Can you work these out from the model? Positions are in its coordinate system, mm. A direction names the side the tool comes from. Round coordinates to 2 decimals unless told otherwise and drop trailing zeros. Loops run counter-clockwise (first coordinate to the right, second up) from the corner with the lowest first, then second, coordinate; pieces in that order, holes last. Notation, with made-up numbers: (-17.75, 65) -> (10.25, 65) arc R9 cw to (10.25, 73) -> close; hole circle Ø11 at (41, 88.5). An arc over 180 degrees is marked (long way). Write each question's results on one line, items separated by ' | '.
from build123d import *

# Parameters (mm, degrees)
F0_W         = 111.7644011974
F0_H         = 111.7644011974
F1_DEPTH     = 55.88
F2_R         = 55.8021322807
F3_R         = 55.8038
F5_T1_DEPTH  = 139.6679689167
F5_T3_DEPTH  = 0.1568011974
F5_T5_DEPTH  = 0.1524
F5_T7_DEPTH  = 139.6679689167
F5_T9_DEPTH  = 0.1568011974
F5_S13_W     = 56.919876
F5_S13_H     = 56.919876
F5_T14_DEPTH = 56.919876
F5_S19_W     = 56.919876
F5_S19_H     = 56.919876
F5_T20_DEPTH = 56.919876
F5_S25_W     = 56.919876
F5_S25_H     = 56.919876
F5_T26_DEPTH = 56.919876
F5_S31_W     = 56.919876
F5_S31_H     = 56.919876
F5_T32_DEPTH = 56.919876
F5_T36_ANGLE = 90
F5_T38_ANGLE = 90
F5_T40_ANGLE = 90
F5_T42_ANGLE = 90
F6_R         = 56.7270748454
F7_DEPTH     = 4.826


# Not quite as in the source:
# - a fillet or chamfer that OpenCascade refuses, or shapes differently, is made with other operations: its cross-section is extruded or revolved along the edge and cut away or added
# - a feature of the source that left no trace in its solid (it failed there, or was rolled back) is left out


with BuildPart() as f1:
    # F0 (on Front) → F1 (new body, symmetric)
    with BuildSketch(Plane.XZ):
        with Locations((-0.1386664808, 0)):
            Rectangle(F0_W, F0_H)
    extrude(amount=F1_DEPTH, both=True)

    # F2
    f2_edges = [f1.edges().sort_by_distance(p)[0] for p in [
        (-56.020867, 0, 55.882201),
    ]]
    fillet(f2_edges, radius=F2_R)

    # F3
    f3_edges = [f1.edges().sort_by_distance(p)[0] for p in [
        (55.743534, 0, 55.882201),
    ]]
    fillet(f3_edges, radius=F3_R)

    # F5: fillet of radius 55.8038 on 10 edges, made by hand

    # F5_s2 → F5_t1 (cut)
    with BuildSketch(Plane.YZ.offset(-139.7282347988)):
        with BuildLine():
            ThreePointArc((0.0762, 55.8822005987), (39.535445396, 39.5376459947), (55.88, 0.0784005987))
            Line((55.88, 0.0784005987), (56.996076, 0.0784005987))
            Line((56.996076, 0.0784005987), (56.996076, 56.9982765987))
            Line((56.996076, 56.9982765987), (0.0762, 56.9982765987))
            Line((0.0762, 56.9982765987), (0.0762, 55.8822005987))
        make_face()
        with BuildLine():
            ThreePointArc((-0.0762, 55.8822005987), (-39.535445396, 39.5376459947), (-55.88, 0.0784005987))
            Line((-55.88, 0.0784005987), (-56.996076, 0.0784005987))
            Line((-56.996076, 0.0784005987), (-56.996076, 56.9982765987))
            Line((-56.996076, 56.9982765987), (-0.0762, 56.9982765987))
            Line((-0.0762, 56.9982765987), (-0.0762, 55.8822005987))
        make_face()
    extrude(amount=F5_T1_DEPTH, mode=Mode.SUBTRACT)

    # F5_s4 → F5_t3 (cut)
    with BuildSketch(Plane.YZ.offset(-0.2170670795)):
        with BuildLine():
            ThreePointArc((55.88, -0.0784005987), (39.535445396, -39.5376459947), (0.0762, -55.8822005987))
            Line((0.0762, -55.8822005987), (0.0762, -56.9982765987))
            Line((0.0762, -56.9982765987), (56.996076, -56.9982765987))
            Line((56.996076, -56.9982765987), (56.996076, -0.0784005987))
            Line((56.996076, -0.0784005987), (55.88, -0.0784005987))
        make_face()
        with BuildLine():
            ThreePointArc((-55.88, -0.0784005987), (-39.535445396, -39.5376459947), (-0.0762, -55.8822005987))
            Line((-0.0762, -55.8822005987), (-0.0762, -56.9982765987))
            Line((-0.0762, -56.9982765987), (-56.996076, -56.9982765987))
            Line((-56.996076, -56.9982765987), (-56.996076, -0.0784005987))
            Line((-56.996076, -0.0784005987), (-55.88, -0.0784005987))
        make_face()
    extrude(amount=F5_T3_DEPTH, mode=Mode.SUBTRACT)

    # F5_s6 → F5_t5 (cut)
    with BuildSketch(Plane.XZ.offset(-0.0762)):
        with BuildLine():
            ThreePointArc((55.7435341179, -0.0784005987), (39.3989795139, -39.5376459947), (-0.0602658821, -55.8822005987))
            Line((-0.0602658821, -55.8822005987), (-0.0602658821, -56.9982765987))
            Line((-0.0602658821, -56.9982765987), (56.8596101179, -56.9982765987))
            Line((56.8596101179, -56.9982765987), (56.8596101179, -0.0784005987))
            Line((56.8596101179, -0.0784005987), (55.7435341179, -0.0784005987))
        make_face()
        with BuildLine():
            ThreePointArc((-56.0208670795, -0.0784005987), (-39.6763124755, -39.5376459947), (-0.2170670795, -55.8822005987))
            Line((-0.2170670795, -55.8822005987), (-0.2170670795, -56.9982765987))
            Line((-0.2170670795, -56.9982765987), (-57.1369430795, -56.9982765987))
            Line((-57.1369430795, -56.9982765987), (-57.1369430795, -0.0784005987))
            Line((-57.1369430795, -0.0784005987), (-56.0208670795, -0.0784005987))
        make_face()
    extrude(amount=F5_T5_DEPTH, mode=Mode.SUBTRACT)

    # F5_s8 → F5_t7 (cut)
    with BuildSketch(Plane.XY.offset(-0.0784005987)):
        with BuildLine():
            ThreePointArc((-0.2170670795, -55.88), (-39.6763124755, -39.535445396), (-56.0208670795, -0.0762))
            Line((-56.0208670795, -0.0762), (-57.1369430795, -0.0762))
            Line((-57.1369430795, -0.0762), (-57.1369430795, -56.996076))
            Line((-57.1369430795, -56.996076), (-0.2170670795, -56.996076))
            Line((-0.2170670795, -56.996076), (-0.2170670795, -55.88))
        make_face()
        with BuildLine():
            ThreePointArc((-0.2170670795, 55.88), (-39.6763124755, 39.535445396), (-56.0208670795, 0.0762))
            Line((-56.0208670795, 0.0762), (-57.1369430795, 0.0762))
            Line((-57.1369430795, 0.0762), (-57.1369430795, 56.996076))
            Line((-57.1369430795, 56.996076), (-0.2170670795, 56.996076))
            Line((-0.2170670795, 56.996076), (-0.2170670795, 55.88))
        make_face()
    extrude(amount=F5_T7_DEPTH, mode=Mode.SUBTRACT)

    # F5_s10 → F5_t9 (cut)
    with BuildSketch(Plane.XY.offset(-0.0784005987)):
        with BuildLine():
            ThreePointArc((-0.0602658821, -55.88), (39.3989795139, -39.535445396), (55.7435341179, -0.0762))
            Line((55.7435341179, -0.0762), (56.8596101179, -0.0762))
            Line((56.8596101179, -0.0762), (56.8596101179, -56.996076))
            Line((56.8596101179, -56.996076), (-0.0602658821, -56.996076))
            Line((-0.0602658821, -56.996076), (-0.0602658821, -55.88))
        make_face()
        with BuildLine():
            ThreePointArc((-0.0602658821, 55.88), (39.3989795139, 39.535445396), (55.7435341179, 0.0762))
            Line((55.7435341179, 0.0762), (56.8596101179, 0.0762))
            Line((56.8596101179, 0.0762), (56.8596101179, 56.996076))
            Line((56.8596101179, 56.996076), (-0.0602658821, 56.996076))
            Line((-0.0602658821, 56.996076), (-0.0602658821, 55.88))
        make_face()
    extrude(amount=F5_T9_DEPTH, mode=Mode.SUBTRACT)


with BuildPart() as f5_tool12:
    # F5_s13 → F5_t14 (new body)
    with BuildSketch(Plane.XZ.offset(-0.0762)):
        with Locations((-28.6770050795, -28.5383385987)):
            Rectangle(F5_S13_W, F5_S13_H)
    extrude(amount=-F5_T14_DEPTH)

    # F5_s15 → F5_t16 (revolve, cut)
    with BuildSketch(Plane(origin=(-0.2170670795, 0.0762, -0.0784005987), x_dir=(0.7071067812, 0, 0.7071067812), z_dir=(-0.7071067812, 0, 0.7071067812))):
        with BuildLine():
            ThreePointArc((0, -55.8038), (55.8038, 0), (0, 55.8038))
            Line((0, 55.8038), (0, -55.8038))
        make_face()
    revolve(axis=Axis((-0.2170670795, 0.0762, -0.0784005987), (0, 1, 0)), mode=Mode.SUBTRACT)


with BuildPart() as f1_1:
    add(f1.part)

    # F5_t11: cut F5_tool12
    add(f5_tool12.part, mode=Mode.SUBTRACT)


with BuildPart() as f5_tool18:
    # F5_s19 → F5_t20 (new body)
    with BuildSketch(Plane.XZ.offset(-0.0762)):
        with Locations((28.3996721179, -28.5383385987)):
            Rectangle(F5_S19_W, F5_S19_H)
    extrude(amount=-F5_T20_DEPTH)

    # F5_s21 → F5_t22 (revolve, cut)
    with BuildSketch(Plane(origin=(-0.0602658821, 0.0762, -0.0784005987), x_dir=(-0.7071067812, 0, 0.7071067812), z_dir=(-0.7071067812, 0, -0.7071067812))):
        with BuildLine():
            ThreePointArc((0, -55.8038), (55.8038, 0), (0, 55.8038))
            Line((0, 55.8038), (0, -55.8038))
        make_face()
    revolve(axis=Axis((-0.0602658821, 0.0762, -0.0784005987), (0, 1, 0)), mode=Mode.SUBTRACT)


with BuildPart() as f1_2:
    add(f1_1.part)

    # F5_t17: cut F5_tool18
    add(f5_tool18.part, mode=Mode.SUBTRACT)


with BuildPart() as f5_tool24:
    # F5_s25 → F5_t26 (new body)
    with BuildSketch(Plane.XZ.offset(0.0762)):
        with Locations((-28.6770050795, -28.5383385987)):
            Rectangle(F5_S25_W, F5_S25_H)
    extrude(amount=F5_T26_DEPTH)

    # F5_s27 → F5_t28 (revolve, cut)
    with BuildSketch(Plane(origin=(-0.2170670795, -0.0762, -0.0784005987), x_dir=(0.7071067812, 0, 0.7071067812), z_dir=(0.7071067812, 0, -0.7071067812))):
        with BuildLine():
            ThreePointArc((0, -55.8038), (55.8038, 0), (0, 55.8038))
            Line((0, 55.8038), (0, -55.8038))
        make_face()
    revolve(axis=Axis((-0.2170670795, -0.0762, -0.0784005987), (0, -1, 0)), mode=Mode.SUBTRACT)


with BuildPart() as f1_3:
    add(f1_2.part)

    # F5_t23: cut F5_tool24
    add(f5_tool24.part, mode=Mode.SUBTRACT)


with BuildPart() as f5_tool30:
    # F5_s31 → F5_t32 (new body)
    with BuildSketch(Plane.XZ.offset(0.0762)):
        with Locations((28.3996721179, -28.5383385987)):
            Rectangle(F5_S31_W, F5_S31_H)
    extrude(amount=F5_T32_DEPTH)

    # F5_s33 → F5_t34 (revolve, cut)
    with BuildSketch(Plane(origin=(-0.0602658821, -0.0762, -0.0784005987), x_dir=(-0.7071067812, 0, 0.7071067812), z_dir=(0.7071067812, 0, 0.7071067812))):
        with BuildLine():
            ThreePointArc((0, -55.8038), (55.8038, 0), (0, 55.8038))
            Line((0, 55.8038), (0, -55.8038))
        make_face()
    revolve(axis=Axis((-0.0602658821, -0.0762, -0.0784005987), (0, -1, 0)), mode=Mode.SUBTRACT)


with BuildPart() as f1_4:
    add(f1_3.part)

    # F5_t29: cut F5_tool30
    add(f5_tool30.part, mode=Mode.SUBTRACT)

    # F5_s35 → F5_t36 (revolve, cut)
    with BuildSketch(Plane.YZ.offset(-0.0602658821)):
        with BuildLine():
            ThreePointArc((55.88, 0.0784005987), (39.535445396, 39.5376459947), (0.0762, 55.8822005987))
            Line((0.0762, 55.8822005987), (0.0762, 56.9982765987))
            Line((0.0762, 56.9982765987), (56.996076, 56.9982765987))
            Line((56.996076, 56.9982765987), (56.996076, 0.0784005987))
            Line((56.996076, 0.0784005987), (55.88, 0.0784005987))
        make_face()
    revolve(axis=Axis((-0.0602658821, 55.88, 0.0784005987), (0, 1, 0)), revolution_arc=F5_T36_ANGLE, mode=Mode.SUBTRACT)

    # F5_s37 → F5_t38 (revolve, cut)
    with BuildSketch(Plane.YZ.offset(-0.2187347988)):
        with BuildLine():
            ThreePointArc((55.8799999751, 0.080068318), (39.5348557638, 39.5382356181), (0.0762, 55.8822005987))
            Line((0.0762, 55.8822005987), (0.0762, 56.9982765987))
            Line((0.0762, 56.9982765987), (56.996076, 56.9982765987))
            Line((56.996076, 56.9982765987), (56.996076, 0.080068318))
            Line((56.996076, 0.080068318), (55.8799999751, 0.080068318))
        make_face()
    revolve(axis=Axis((-0.2187347988, 55.88, 0.080068318), (0, -1, 0)), revolution_arc=F5_T38_ANGLE, mode=Mode.SUBTRACT)

    # F5_s39 → F5_t40 (revolve, cut)
    with BuildSketch(Plane.YZ.offset(-0.0602658821)):
        with BuildLine():
            ThreePointArc((-0.0762, 55.8822005987), (-39.535445396, 39.5376459947), (-55.88, 0.0784005987))
            Line((-55.88, 0.0784005987), (-56.996076, 0.0784005987))
            Line((-56.996076, 0.0784005987), (-56.996076, 56.9982765987))
            Line((-56.996076, 56.9982765987), (-0.0762, 56.9982765987))
            Line((-0.0762, 56.9982765987), (-0.0762, 55.8822005987))
        make_face()
    revolve(axis=Axis((-0.0602658821, -55.88, 0.0784005987), (0, 1, 0)), revolution_arc=F5_T40_ANGLE, mode=Mode.SUBTRACT)

    # F5_s41 → F5_t42 (revolve, cut)
    with BuildSketch(Plane.YZ.offset(-0.2187347988)):
        with BuildLine():
            ThreePointArc((-0.0762, 55.8822005987), (-39.5348557638, 39.5382356181), (-55.8799999751, 0.080068318))
            Line((-55.8799999751, 0.080068318), (-56.996076, 0.080068318))
            Line((-56.996076, 0.080068318), (-56.996076, 56.9982765987))
            Line((-56.996076, 56.9982765987), (-0.0762, 56.9982765987))
            Line((-0.0762, 56.9982765987), (-0.0762, 55.8822005987))
        make_face()
    revolve(axis=Axis((-0.2187347988, -55.88, 0.080068318), (0, -1, 0)), revolution_arc=F5_T42_ANGLE, mode=Mode.SUBTRACT)

    # F6 (on Top) → F7 (join, symmetric)
    with BuildSketch(Plane.XY):
        Circle(F6_R)
    extrude(amount=F7_DEPTH, both=True)


solid = f1_4.part
1. If we section it at B-B (x = 28): List the corners of the cut face in (y, z) for me, then the cut area to 3 significant figures.
Final values:
outline: (-49.34, -4.83) -> (-48.08, -4.83) arc R48.24 ccw to (-0.08, -48.31) -> (0.08, -48.31) arc R48.24 ccw to (48.08, -4.83) -> (49.34, -4.83) -> (49.34, 4.83) -> (48.08, 4.83) arc R48.24 ccw to (0.08, 48.31) -> (-0.08, 48.31) arc R48.24 ccw to (-48.08, 4.83) -> (-49.34, 4.83) -> close | area: 7,360 mm2
2. Please list where these lines run through material, in increasing order: line 1 (X direction, y = 37.5, z = 35.5); line 2 (X direction, y = -34, z = -8.5); line 3 (Z direction, x = 17.5, y = -25). Write a range as from..to.
Final values:
line 1: -21.64..21.36 | line 2: -43.72..43.44 | line 3: -46.82..46.82
3. Will these pins go through, and if not, where does the flat tip stop? pin 1 (1 mm diameter, centred on x = -31, y = 26, fed in from +Z); pin 2 (10 mm diameter, centred on x = -13, z = -29.5, fed in from +Y); pin 3 (3 mm diameter, centred on x = -9, z = -10.5, fed in from +Y).
Final values:
pin 1: z = 39.25 | pin 2: y = 48.87 | pin 3: y = 54.55
4. If we section it at A-A (z = -21): List the corners of the cut face in (x, y) for me, then the cut area to 3 significant figures.
Final values:
outline: (-51.95, -0.08) arc R51.73 ccw to (-0.22, -51.81) -> (-0.06, -51.81) arc R51.73 ccw to (51.67, -0.08) -> (51.67, 0.08) arc R51.73 ccw to (-0.06, 51.81) -> (-0.22, 51.81) arc R51.73 ccw to (-51.95, 0.08) -> close | area: 8,440 mm2
5. On a 3-axis mill with a long thin cutter (end or side, diameter ignored), from which of +Z, -Z, +X, -X, +Y, -Y can I reach the whole of each face in a straight line? I mean faces 1 (the face through (41.8, -37.6, 4.826)), 2 (the face through (41.8, -37.6, -4.826)), 3 (the face through (52.4, -21.73, 0.07)). Say none if no direction works.
Final values:
face 1: +Z | face 2: -Z | face 3: +Z, -Z
6. If we section it at C-C (z = 2.5): List the corners of the cut face in (x, y) for me.
Final values:
outline: circle Ø113.45 at (0, 0)
